Autodesk Inventor part; units mm, degrees
ref_plane "YZ Plane" through (0, 0, 0) normal (1, 0, 0) x (0, 1, 0)
ref_plane "XZ Plane" through (0, 0, 0) normal (0, 1, 0) x (-1, 0, 0)
ref_plane "XY Plane" through (0, 0, 0) normal (0, 0, 1) x (1, 0, 0)
sketch "Эскиз1" plane through (0, 0, 0) normal (0, 1, 0) x (-1, 0, 0)
  line L0 (0, -45) -> (-38.9711, -22.5)
  line L1 (-38.9711, -22.5) -> (-38.9711, 22.5)
  line L2 (-38.9711, 22.5) -> (0, 45)
  line L3 (0, 45) -> (38.9711, 22.5)
  line L4 (38.9711, 22.5) -> (38.9711, -22.5)
  line L5 (38.9711, -22.5) -> (0, -45)
  point P0 (0, 0)
  point P1 (0, 0)
  dimension "d2" = 45
extrude "Выдавливание1" add sketch "Эскиз1" along normal blind 45
sketch "Эскиз3" plane through (0, 0, 0) normal (1, 0, 0) x (0, 1, 0)
  line L0 (45, -22.5) -> (45, 22.5)
  line L1 (45, 0) -> (80, 0)
  line L2 (45, 22.5) -> (45, -22.5)
  line L3 (45, 0) -> (45, -35)
  arc A0 (45, -35) -> (45, 35) centre (45, 0) ccw
  point P0 (0, 0)
  dimension "d3" = 35
  dimension "d4" = 35
revolve "Вращение1" add sketch "Эскиз3" angle 360 about axis through (0, 45, 0) along (0, 1, 0)
sketch "Эскиз5" plane through (0, 0, 0) normal (1, 0, 0) x (0, 1, 0)
  arc A0 (45, -35) -> (45, 35) centre (45, 0) ccw
  line L0 (0, 22.5) -> (0, 45)
  line L1 (77.2198, 45) -> (0, 45)
  line L2 (97.7076, -23.3946) -> (97.7076, 45.0272)
  line L3 (97.7076, 45.0272) -> (76.0865, 45)
  line L4 (97.7076, -23.3946) -> (0, 45)
  point P0 (0, 0)
  point P1 (78.541, -10)
  point P2 (80, 0)
  dimension "d6" = 10
extrude "Выдавливание2" cut sketch "Эскиз5" along normal blind 100 and the other way blind 100
Check sheet for the modelled part. Datum: model origin and axes. Units: mm. Coordinates: 2 decimals unless noted, no trailing zeros. Write each loop counter-clockwise with the first axis right and the second up, starting at its lowest first coordinate (ties: lowest second). Pieces come first, ordered by that corner, then holes. Notation, with made-up numbers: (41, -15) -> (62, -15) arc R30 cw to (62, 17) -> close; hole circle Ø8 at (-32, 73). An arc over 180 degrees is marked (long way). Use a Markdown table: item, result.
1. Scan lines: line 1 along Y through (x, z) = (35, -24); line 2 along Z through (x, y) = (-10, 60); line 3 along Z through (x, y) = (-21.5, 18). Record each from-to range of solid material in increasing order.
Reported:
| item | result |
|---|---|
| line 1 | y = 0 to 45 |
| line 2 | z = -30 to 3 |
| line 3 | z = -32.59 to 32.4 |
2. Sectioned sample at B-B (z = -21). Enter the section's corners in (x, y), plus the area to 3 significant figures.
Reported:
| item | result |
|---|---|
| outline | (-38.97, 0) -> (38.97, 0) -> (38.97, 45) -> (28, 45) arc R28 ccw to (-28, 45) -> (-38.97, 45) -> close |
| area | 4,740 mm2 |
3. Sectioned sample at D-D (y = 41.5). Enter the section's corners in (x, z), plus the area to 3 significant figures.
Reported:
| item | result |
|---|---|
| outline | (-38.97, -22.5) -> (0, -45) -> (38.97, -22.5) -> (38.97, 15.95) -> (-38.97, 15.95) -> close |
| area | 3,870 mm2 |
4. Sectioned sample at A-A (y = 30). Enter the section's corners in (x, z), plus the area to 3 significant figures.
Reported:
| item | result |
|---|---|
| outline | (-38.97, -22.5) -> (0, -45) -> (38.97, -22.5) -> (38.97, 22.5) -> (36.37, 24) -> (-36.37, 24) -> (-38.97, 22.5) -> close |
| area | 4,500 mm2 |
5. Go/stop test with flat-tipped pins: pin 1 Ø2 at (x, y) = (21, 65.5) entering from -Z; pin 2 Ø5 at (x, y) = (11, 70.5) entering from +Z; pin 3 Ø2 at (x, y) = (-11.5, 44) entering from -Z. Record where each tip stops, or that it passes through.
Reported:
| item | result |
|---|---|
| pin 1 | stops at z = -20.53 |
| pin 2 | stops at z = -2.6 |
| pin 3 | stops at z = -38.94 |
6. Sectioned sample at C-C (x = 16). Enter the section's corners in (y, z), plus the area to 3 significant figures.
Reported:
| item | result |
|---|---|
| outline | (0, -35.76) -> (45, -35.76) -> (45, -31.13) arc R31.13 ccw to (75.18, -7.63) -> (13.2, 35.76) -> (0, 35.76) -> close |
| area | 3,710 mm2 |
